from build123d import *

# Parameters (mm, degrees)
BOSS_EXTRUDE1_DEPTH = 3
SKETCH2_R           = 1.6
CUT_EXTRUDE1_DEPTH  = 69.571130952
CHAMFER1_SIZE       = 1.5


with BuildPart() as part:
    # Sketch1 → Boss-Extrude1 (new body)
    with BuildSketch(Plane(origin=(0, 0, 0), x_dir=(1, 0, 0), z_dir=(0, 1, 0))):
        Polygon((0, -57), (-35, -57), (-35, -37), (-38, -37), (-38, -12), (-35, -12), (-35, 12), (-38, 12), (-38, 37), (-35, 37), (-35, 52), (-12.666666667, 52), (-12.666666667, 57), (0, 57), align=None)
    boss_extrude1 = extrude(amount=BOSS_EXTRUDE1_DEPTH)

    # Mirror1: Boss-Extrude1 across plane
    add(boss_extrude1.mirror(Plane(origin=(0, 3, -57), x_dir=(0, 0, 1), z_dir=(-1, 0, 0))))

    # Sketch2 → Cut-Extrude1 (cut, through all)
    with BuildSketch(Plane(origin=(0, 3, 0), x_dir=(1, 0, 0), z_dir=(0, 1, 0))):
        with Locations(Location((-25.5, 5, 0), (0, 0, 270))):
            Circle(SKETCH2_R)
        with Locations(Location((25.5, 5, 0), (0, 0, 270))):
            Circle(SKETCH2_R)
    extrude(amount=-CUT_EXTRUDE1_DEPTH, mode=Mode.SUBTRACT)

    # Chamfer1
    chamfer1_edges = [part.edges().sort_by_distance(p)[0] for p in [
        (-25.5, 3, -6.6),
        (25.5, 3, -6.6),
    ]]
    chamfer(chamfer1_edges, length=CHAMFER1_SIZE)


solid = part.part
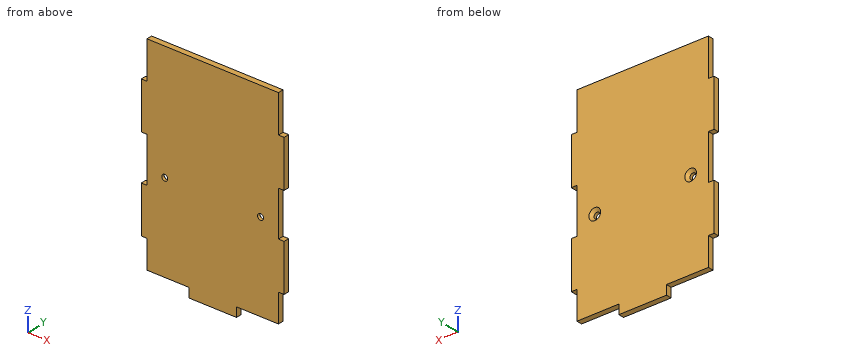
The model under review builds one solid part; all positions refer to its coordinate system, in mm. Coordinates: 2 decimals unless noted, no trailing zeros. Write each loop counter-clockwise with the first axis right and the second up, starting at its lowest first coordinate (ties: lowest second). Pieces come first, ordered by that corner, then holes. Notation, with made-up numbers: (54.25, 23.5) -> (106.25, 23.5) arc R32 cw to (106.25, 49.5) -> close; hole circle Ø9 at (37, 85.25). An arc over 180 degrees is marked (long way). Answer in a Markdown table with one row per item.
1. We need section A-A, the plane y = 2.55. State the section outline as (x, z) points.
Answers below:
| item | result |
|---|---|
| outline | (-38, -37) -> (-35, -37) -> (-35, -52) -> (-12.67, -52) -> (-12.67, -57) -> (12.67, -57) -> (12.67, -52) -> (35, -52) -> (35, -37) -> (38, -37) -> (38, -12) -> (35, -12) -> (35, 12) -> (38, 12) -> (38, 37) -> (35, 37) -> (35, 57) -> (-35, 57) -> (-35, 37) -> (-38, 37) -> (-38, 12) -> (-35, 12) -> (-35, -12) -> (-38, -12) -> close; hole circle Ø5.3 at (-25.5, -5); hole circle Ø5.3 at (25.5, -5) |
2. Clearance check with flat-ended pins moving along their axes: pin 1 Ø0.9 at (y, z) = (1.5, -6) entering from +X; pin 2 Ø1.5 at (y, z) = (1, -53.5) entering from -X; pin 3 Ø1 at (x, y) = (23, 2.5) entering from -Z; pin 4 Ø6 at (x, z) = (-5.5, -15) entering from -Y. State where each tip first meets the part, or that it passes through.
Answers below:
| item | result |
|---|---|
| pin 1 | stops at x = 35 |
| pin 2 | stops at x = -12.67 |
| pin 3 | stops at z = -52 |
| pin 4 | stops at y = 0 |
3. We need section C-C, the plane z = -5. State the section outline as (x, y) points.
Answers below:
| item | result |
|---|---|
| outline | (-35, 0) -> (-27.1, 0) -> (-27.1, 1.5) -> (-28.6, 3) -> (-35, 3) -> close; (-23.9, 0) -> (23.9, 0) -> (23.9, 1.5) -> (22.4, 3) -> (-22.4, 3) -> (-23.9, 1.5) -> close; (27.1, 0) -> (35, 0) -> (35, 3) -> (28.6, 3) -> (27.1, 1.5) -> close |
4. We need section D-D, the plane z = 46. State the section outline as (x, y) points.
Answers below:
| item | result |
|---|---|
| outline | (-35, 0) -> (35, 0) -> (35, 3) -> (-35, 3) -> close |
5. We need section B-B, the plane x = -25.5. State the section outline as (y, z) points.
Answers below:
| item | result |
|---|---|
| outline | (0, -52) -> (3, -52) -> (3, -8.1) -> (1.5, -6.6) -> (0, -6.6) -> close; (0, -3.4) -> (1.5, -3.4) -> (3, -1.9) -> (3, 57) -> (0, 57) -> close |
6. Wall thickness on probe 1 along X at (y, z) = (0.65, -5); probe 2 along Z at (x, y) = (-21.5, 1.55); probe 3 along X at (y, z) = (0.95, 43): over which ranges is each line inside the solid? List them lowest first. Write a range as [from, to].
Answers below:
| item | result |
|---|---|
| probe 1 | x = [-35, -27.1], [-23.9, 23.9], [27.1, 35] |
| probe 2 | z = [-52, 57] |
| probe 3 | x = [-35, 35] |
